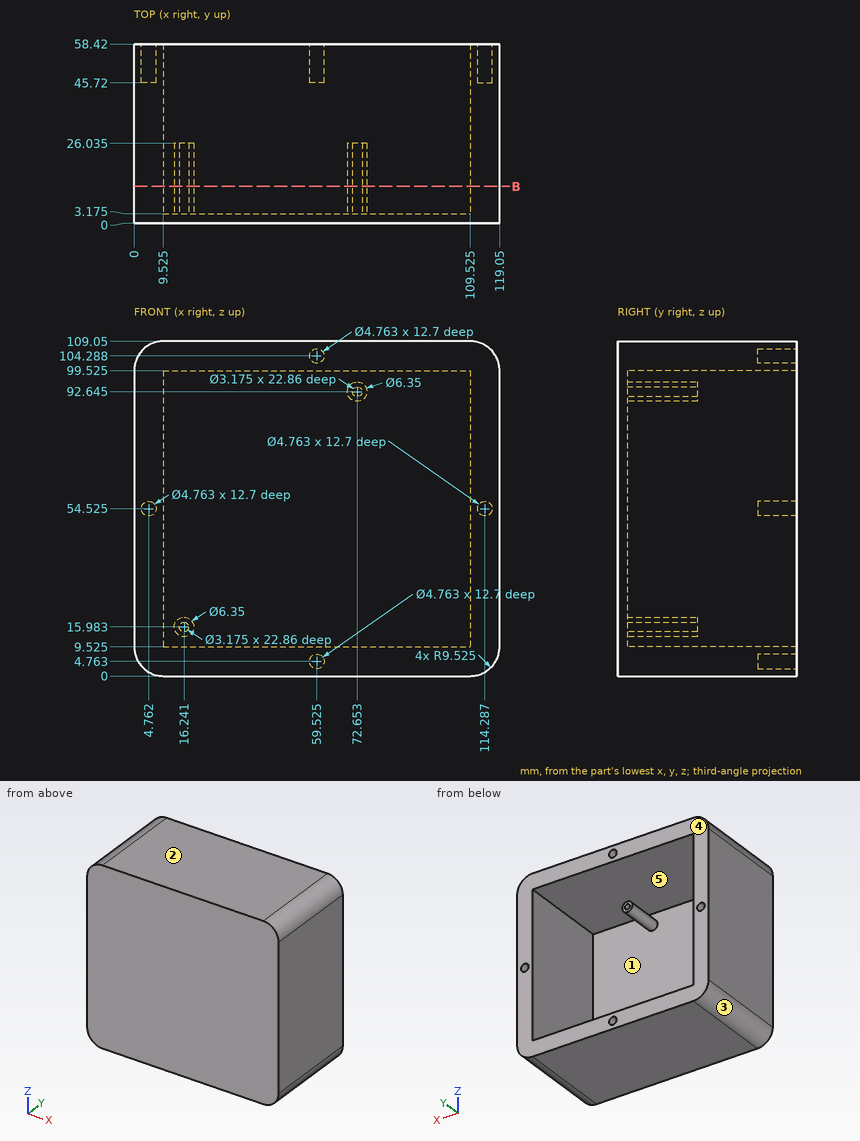
Here's the drawing with two shaded views (mm, measured from the low corner). I have some questions. A direction names the side the tool comes from. Coordinates: 2 decimals unless noted, no trailing zeros. Put each result on its own line as item: value. Start each with the question number.
(1) Will these pins go through, and if not, where does the flat tip stop? pin 1 Ø1.4 at (x, z) = (60.5, 4.5) entering from +Y; pin 2 Ø3 at (x, z) = (73, 93) entering from +Y (1 decimal); pin 3 Ø1 at (x, z) = (16.5, 16.5) entering from +Y (1 decimal).
(2) Imagine slicing it at B-B on y = 12. Give the number of separate pieces and of enclosed holes in the cut face, and give its area (3 significant figures).
(3) I need wall thicknesses on probe 1 along Y at (x, z) = (62, 27) (1 decimal); probe 2 along Y at (x, z) = (17.5, 17) (1 decimal); probe 3 along X at (y, z) = (33.5, 7). Which ranges of each line are inside material? Lowest first, please.
(4) We'd pull the mould along X, two halves only. Please class the marked faces 3, 4 and 5: +X half, -X half, draft (parallel to the pull), parting line (faces both ways), or undercut.
(5) Which directions (+Z, -Z, +X, -X, +Y, -Y) give clear straight access to the entire face, cutting with the end or side of a thin tool? Please do the marked faces 1 and 2.
Worked answers:
1. pin 1: stops at y = 45.72
1. pin 2: stops at y = 26
1. pin 3: stops at y = 3.2
2. separate pieces: 3
2. enclosed holes: 3
2. area: 3,950 mm2
3. probe 1: y = 0 to 3.2
3. probe 2: y = 0 to 26
3. probe 3: x = 0.34 to 118.71
4. face 3: -X half
4. face 4: draft
4. face 5: undercut
5. face 1: +Y
5. face 2: +Z, +X, -X, +Y, -Y
